from build123d import *

# Parameters (mm, degrees)
SKETCH1_W           = 31.75
SKETCH1_H           = 15
BOSS_EXTRUDE1_DEPTH = 8
SKETCH2_W           = 5
SKETCH2_H           = 15
BOSS_EXTRUDE2_DEPTH = 69.1
SKETCH3_R           = 2.5
CUT_EXTRUDE1_DEPTH  = 69.1
SKETCH4_R           = 4
SKETCH4_R_2         = 2
CUT_EXTRUDE3_DEPTH  = 4
SKETCH5_R           = 1.5
CUT_EXTRUDE4_DEPTH  = 3
SKETCH6_R           = 1.5
CUT_EXTRUDE5_DEPTH  = 37


with BuildPart() as part:
    # Sketch1 → Boss-Extrude1 (new body)
    with BuildSketch(Plane.XY):
        with Locations((-0.926352113, 0.669031185)):
            Rectangle(SKETCH1_W, SKETCH1_H)
    extrude(amount=BOSS_EXTRUDE1_DEPTH)

    # Sketch2 → Boss-Extrude2 (add)
    with BuildSketch(Plane.XY.offset(8)):
        with Locations((-14.301352113, 0.669031185)):
            Rectangle(SKETCH2_W, SKETCH2_H)
        with Locations((12.448647887, 0.669031185)):
            Rectangle(SKETCH2_W, SKETCH2_H)
    extrude(amount=BOSS_EXTRUDE2_DEPTH)

    # Sketch3 → Cut-Extrude1 (cut)
    with BuildSketch(Plane(origin=(14.948647887, 0, 0), x_dir=(0, 0, -1), z_dir=(1, 0, 0))):
        with Locations(Location((-66.1, 0.669031185, 0), (0, 0, 90))):
            Circle(SKETCH3_R)
    extrude(amount=-CUT_EXTRUDE1_DEPTH, mode=Mode.SUBTRACT)

    # Sketch4 → Cut-Extrude3 (cut)
    with BuildSketch(Plane(origin=(0, 0, 0), x_dir=(-1, 0, 0), z_dir=(0, 0, -1))):
        with Locations((0.926352113, 0.669031185)):
            Circle(SKETCH4_R)
        with Locations((0.926352113, 0.669031185)):
            Circle(SKETCH4_R_2, mode=Mode.SUBTRACT)
    extrude(amount=-CUT_EXTRUDE3_DEPTH, mode=Mode.SUBTRACT)

    # Sketch5 → Cut-Extrude4 (cut)
    with BuildSketch(Plane.XZ.offset(6.830968815)):
        with Locations((-0.926352113, 4)):
            Circle(SKETCH5_R)
    extrude(amount=-CUT_EXTRUDE4_DEPTH, mode=Mode.SUBTRACT)

    # Sketch6 → Cut-Extrude5 (cut)
    with BuildSketch(Plane(origin=(14.948647887, 0, 0), x_dir=(0, 0, -1), z_dir=(1, 0, 0))):
        with Locations(Location((-74.6, 0.669031185, 0), (0, 0, 90))):
            Circle(SKETCH6_R)
    extrude(amount=-CUT_EXTRUDE5_DEPTH, mode=Mode.SUBTRACT)


solid = part.part
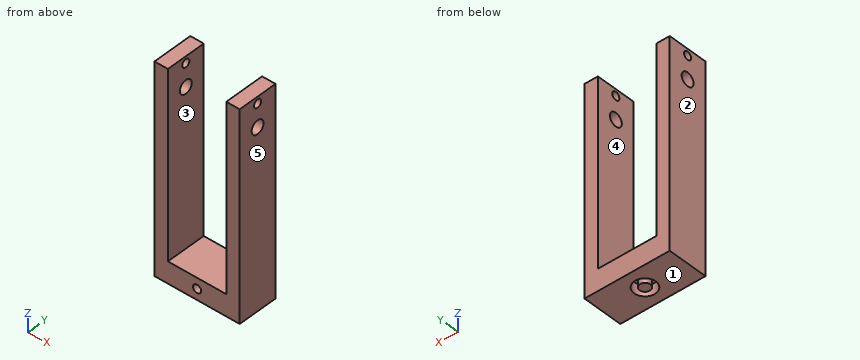
Input: part model. Units: mm. Frame: model coordinates. Face numbers are marked on the shaded views. A direction names the side the tool comes from. Give positions to 0.01 mm unless a question says otherwise; leave off trailing zeros. Loops run counter-clockwise (first coordinate to the right, second up) from the corner with the lowest first, then second, coordinate; pieces in that order, holes last. Notation, with made-up numbers: (-36.75, 64.25) -> (-20.75, 64.25) arc R20 cw to (-20.75, 78.25) -> close; hole circle Ø3 at (72, -7). An arc over 180 degrees is marked (long way). Answer as a JSON object with one key per item and string values. Group by question number.
Item 1: Cut plane C-C, the plane x = 11.5. Return the cut outline in (y, z), and give its area (3 significant figures).
Item 2: Cut plane D-D, the plane y = 6.5. Return the cut outline in (x, z).
Item 3: Cut plane A-A, the plane z = 74.6. Return the cut outline in (x, y).
Item 4: Pin query (flat end, axial travel): P1, Ø1.8, axis at x = -0.93, z = 4, coming from the -Y side; P2, Ø7.5, axis at x = 2.5, y = -1.5, coming from the +Z side; P3, Ø1, axis at x = -4, y = -0.5, coming from the -Z side. Return the tip coordinate at first contact, or that it passes through.
Item 5: Pull-direction query (X, two-part tool) for the marked faces 1, 2 and 3; classes: released by +X, released by -X, zero draft, split by the parting line, or undercut.
Item 6: Line query: probe 1 along X at (y, z) = (-2.25, 52.5); probe 2 along Y at (x, z) = (13.5, 74.6); probe 3 along Z at (x, y) = (8, -3.75). Output: solid intervals per line, ascending.
Item 7: Cut plane B-B, the plane z = 26. Return the cut outline in (x, y).
Item 8: Reachability of the marked faces 4 and 5 from +Z, -Z, +X, -X, +Y, -Y: full face, straight path, thin tool, end or side. Return the list, or none.
Checks:
{
 "1": {"outline": "(-6.83, 0) -> (8.17, 0) -> (8.17, 77.1) -> (-6.83, 77.1) -> close; hole circle Ø5 at (0.67, 66.1); hole circle Ø3 at (0.67, 74.6)", "area": "1,130 mm²"},
 "2": {"outline": "(-16.8, 0) -> (14.95, 0) -> (14.95, 77.1) -> (9.95, 77.1) -> (9.95, 8) -> (-11.8, 8) -> (-11.8, 77.1) -> (-16.8, 77.1) -> close"},
 "3": {"outline": "(-16.8, -6.83) -> (-11.8, -6.83) -> (-11.8, -0.83) -> (-16.8, -0.83) -> close; (-16.8, 2.17) -> (-11.8, 2.17) -> (-11.8, 8.17) -> (-16.8, 8.17) -> close; (9.95, -6.83) -> (14.95, -6.83) -> (14.95, -0.83) -> (9.95, -0.83) -> close; (9.95, 2.17) -> (14.95, 2.17) -> (14.95, 8.17) -> (9.95, 8.17) -> close"},
 "4": {"P1": "stops at y = -3.83", "P2": "stops at z = 8", "P3": "stops at z = 4"},
 "5": {"face 1": "zero draft", "face 2": "released by -X", "face 3": "undercut"},
 "6": {"probe 1": "x = -16.8 to -11.8, 9.95 to 14.95", "probe 2": "y = -6.83 to -0.83, 2.17 to 8.17", "probe 3": "z = 0 to 8"},
 "7": {"outline": "(-16.8, -6.83) -> (-11.8, -6.83) -> (-11.8, 8.17) -> (-16.8, 8.17) -> close; (9.95, -6.83) -> (14.95, -6.83) -> (14.95, 8.17) -> (9.95, 8.17) -> close"},
 "8": {"face 4": "+Z, +Y, -Y", "face 5": "+Z, -Z, +X, +Y, -Y"}
}
